For this review, take the finished solid that the model builds, in its own axes (mm). Face numbers are marked on the shaded views. A direction names the side the tool comes from. Coordinates: 2 decimals unless noted, no trailing zeros. Write each loop counter-clockwise with the first axis right and the second up, starting at its lowest first coordinate (ties: lowest second). Pieces come first, ordered by that corner, then holes. Notation, with made-up numbers: M 47.5,21.5 L 65.5,21.5 A25 ccw 65.5,60.5 Z; hole C 19.5,38 d11. An arc over 180 degrees is marked long. One line per question, with ' | ' between items.
from build123d import *

# Parameters (mm, degrees)
BOSS_EXTRUDE1_DEPTH = 3
SKETCH2_R           = 4.25
CUT_EXTRUDE1_DEPTH  = 3
SKETCH3_R           = 1.75
CUT_EXTRUDE2_DEPTH  = 3


with BuildPart() as part:
    # Sketch1 → Boss-Extrude1 (new body)
    with BuildSketch(Plane.XY):
        with BuildLine():
            Line((-17, 12.5), (17, 12.5))
            ThreePointArc((17, 12.5), (19.121320344, 11.621320344), (20, 9.5))
            Line((20, 9.5), (20, -9.5))
            ThreePointArc((20, -9.5), (19.121320344, -11.621320344), (17, -12.5))
            Line((17, -12.5), (-17, -12.5))
            ThreePointArc((-17, -12.5), (-19.121320344, -11.621320344), (-20, -9.5))
            Line((-20, -9.5), (-20, 9.5))
            ThreePointArc((-20, 9.5), (-19.121320344, 11.621320344), (-17, 12.5))
        make_face()
    extrude(amount=BOSS_EXTRUDE1_DEPTH)

    # Sketch2 → Cut-Extrude1 (cut)
    with BuildSketch(Plane.XY.offset(3)):
        with Locations((-5.25, 5.27)):
            Circle(SKETCH2_R)
        with Locations((5.25, 5.27)):
            Circle(SKETCH2_R)
        with BuildLine():
            Line((-9.5, -4.73), (-9.5, -8.98))
            Line((-9.5, -8.98), (-1, -8.98))
            Line((-1, -8.98), (-1, -4.73))
            ThreePointArc((-1, -4.73), (-5.25, -0.48), (-9.5, -4.73))
        make_face()
        with BuildLine():
            Line((1, -4.73), (1, -8.98))
            Line((1, -8.98), (9.5, -8.98))
            Line((9.5, -8.98), (9.5, -4.73))
            ThreePointArc((9.5, -4.73), (5.25, -0.48), (1, -4.73))
        make_face()
    extrude(amount=-CUT_EXTRUDE1_DEPTH, mode=Mode.SUBTRACT)

    # Sketch3 → Cut-Extrude2 (cut)
    with BuildSketch(Plane.XY.offset(3)):
        with Locations((-15, 0)):
            Circle(SKETCH3_R)
        with Locations((15, 0)):
            Circle(SKETCH3_R)
    extrude(amount=-CUT_EXTRUDE2_DEPTH, mode=Mode.SUBTRACT)


solid = part.part
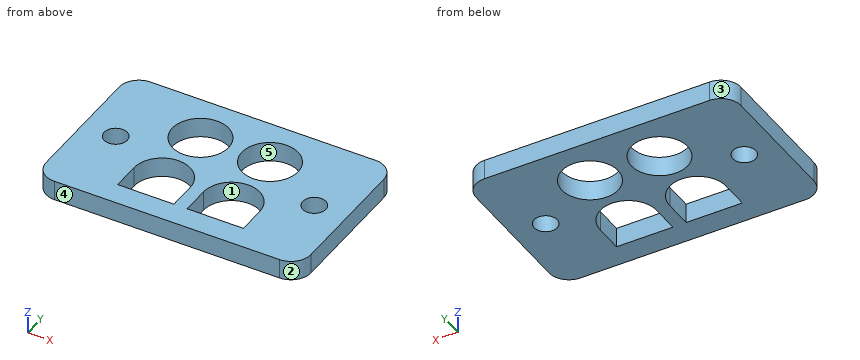
1) We need section D-D on x = -15. State the section outline as (y, z) points.
Responses:
outline: M -12.5,0 L -1.75,0 L -1.75,3 L -12.5,3 Z; M 1.75,0 L 12.5,0 L 12.5,3 L 1.75,3 Z
2) We need section A-A on x = -5.25. State the section outline as (y, z) points.
Responses:
outline: M -12.5,0 L -8.98,0 L -8.98,3 L -12.5,3 Z; M -0.48,0 L 1.02,0 L 1.02,3 L -0.48,3 Z; M 9.52,0 L 12.5,0 L 12.5,3 L 9.52,3 Z
3) The part is to be moulded in two halves that separate along X. For the marked faces 3, 4 and 5, say which applies: +X half, -X half, draft (parallel to the pull), parting line (faces both ways), or undercut.
Responses:
face 3: -X half | face 4: draft | face 5: undercut
4) To check wall thickness, follow line 1 along Y through (x, z) = (-5.25, 2.2); line 2 along X through (y, z) = (-5.5, 1.55); line 3 along X through (y, z) = (-0.25, 1.1). State the ranges of each line that lie inside material, in increasing order. Write a range as [from, to].
Responses:
line 1: [-12.5, -8.98], [-0.48, 1.02], [9.52, 12.5] | line 2: [-20, -9.5], [-1, 1], [9.5, 20] | line 3: [-20, -16.73], [-13.27, 13.27], [16.73, 20]
5) We need section B-B on y = -5.25. State the section outline as (x, z) points, then the cut area to 3 significant figures.
Responses:
outline: M -20,0 L -9.5,0 L -9.5,3 L -20,3 Z; M -1,0 L 1,0 L 1,3 L -1,3 Z; M 9.5,0 L 20,0 L 20,3 L 9.5,3 Z | area: 69.0 mm^2
6) Machinability: for the marked faces 1 and 2, which of the approach directions +Z, -Z, +X, -X, +Y, -Y give a long, thin tool a straight path to every point of the face, cutting with its end or side? Answer none if there is none.
Responses:
face 1: +Z, -Z | face 2: +Z, -Z, +X, -Y
7) We need section C-C on z = 1.6. State the section outline as (x, y) points, then the cut area to 3 significant figures.
Responses:
outline: M -20,-9.5 A3 ccw -17,-12.5 L 17,-12.5 A3 ccw 20,-9.5 L 20,9.5 A3 ccw 17,12.5 L -17,12.5 A3 ccw -20,9.5 Z; hole C -15,0 d3.5; hole M -9.5,-8.98 L -1,-8.98 L -1,-4.73 A4.25 ccw -9.5,-4.73 Z; hole C -5.25,5.27 d8.5; hole M 1,-8.98 L 9.5,-8.98 L 9.5,-4.73 A4.25 ccw 1,-4.73 Z; hole C 5.25,5.27 d8.5; hole C 15,0 d3.5 | area: 731 mm^2
